Could you check a few things on this drawing? It's one solid part, dimensions in mm from its lowest x, y, z. Round coordinates to 2 decimals unless told otherwise and drop trailing zeros. Loops run counter-clockwise (first coordinate to the right, second up) from the corner with the lowest first, then second, coordinate; pieces in that order, holes last. Notation, with made-up numbers: (80.5, 45.25) -> (135.5, 45.25) arc R18 cw to (135.5, 51.25) -> close; hole circle Ø10 at (-36, 44). An arc over 180 degrees is marked (long way). Write each question's results on one line, items separated by ' | '.
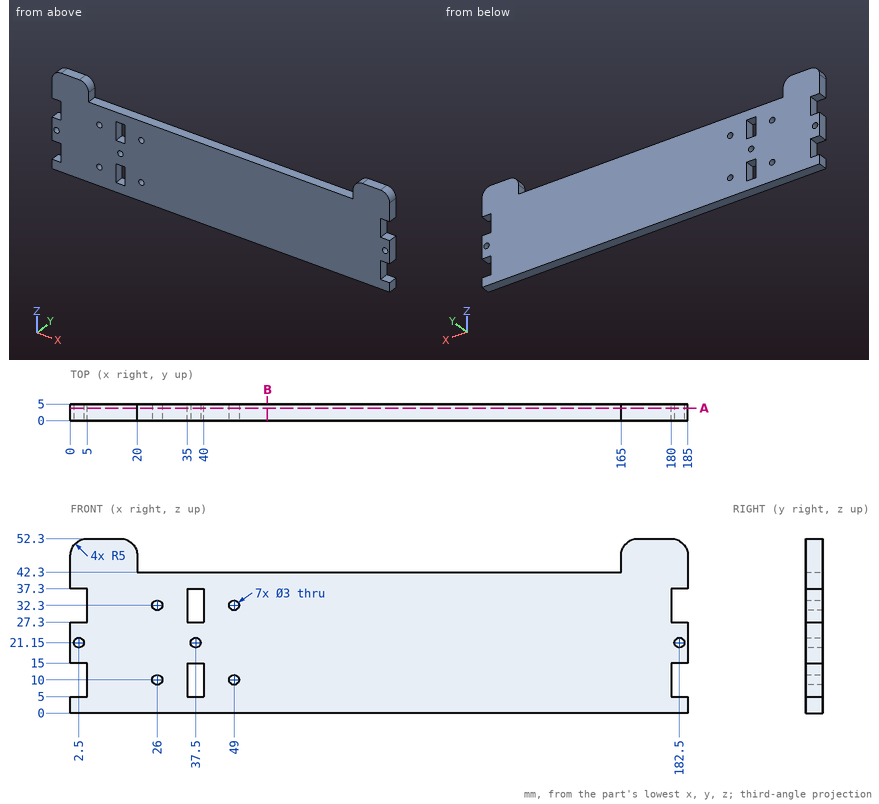
1) I want a section at B-B, the plane x = 59. Write out the boundary of the cut face in (y, z).
Model answer:
outline: (0, 0) -> (5, 0) -> (5, 42.3) -> (0, 42.3) -> close
2) I need wall thicknesses on line 1 (X direction, y = 2.2, z = 32.3); line 2 (X direction, y = 1.3, z = 21.15); line 3 (Z direction, x = 39.5, y = 4.8). Which ranges of each line are inside material? Lowest first, please.
Model answer:
line 1: x = 5 to 24.5, 27.5 to 35, 40 to 47.5, 50.5 to 180 | line 2: x = 0 to 1, 4 to 36, 39 to 181, 184 to 185 | line 3: z = 0 to 5, 15 to 27.3, 37.3 to 42.3
3) I'm going to push flat-ended pins straight in: pin 1 (1.5 mm diameter, centred on y = 1.5, z = 31.5, fed in from +X); pin 2 (2.5 mm diameter, centred on x = 183, y = 3, fed in from +Z); pin 3 (1.5 mm diameter, centred on y = 3, z = 8, fed in from -X). Where does each tip first touch, or does it pass through?
Model answer:
pin 1: stops at x = 180 | pin 2: stops at z = 51.98 | pin 3: stops at x = 5
4) I want a section at A-A, the plane y = 3.75. Give the number of separate pieces and of enclosed holes in the cut face, plus the area to 3 significant figures.
Model answer:
separate pieces: 1 | enclosed holes: 9 | area: 7,850 mm2
